Design review of the part built by this model. Coordinates are the model's own, in mm. Face numbers are marked on the shaded views. A direction names the side the tool comes from. Round coordinates to 2 decimals unless told otherwise and drop trailing zeros. Loops run counter-clockwise (first coordinate to the right, second up) from the corner with the lowest first, then second, coordinate; pieces in that order, holes last. Notation, with made-up numbers: (41.25, -33) -> (100.25, -33) arc R29 cw to (100.25, -8) -> close; hole circle Ø1 at (76.5, -1.5). An arc over 180 degrees is marked (long way). Answer as CSV lines item,"result". Start each with the question number.
(1) Machinability: for the marked faces 4, 5, 6, 7 and 8, which of the approach directions +Z, -Z, +X, -X, +Y, -Y give a long, thin tool a straight path to every point of the face, cutting with its end or side? Answer none if there is none.
(2) Take a section at C-C, the plane z = -15.5. Write out the cut boundary in (x, y), and give its area (4 significant figures).
(3) Draft analysis for pull direction Z (two halves, no side actions). For the marked faces 1, 2 and 3, state which applies: +Z half, -Z half, draft (parallel to the pull), parting line (faces both ways), or undercut.
(4) Take a section at A-A, the plane y = 54.5. Write out the cut boundary in (x, z), and give its area (3 significant figures).
(5) To check wall thickness, follow line 1 (Z direction, x = 24, y = 43); line 2 (X direction, y = 4, z = 28.5); line 3 (Z direction, x = 54, y = 28). State the ranges of each line that lie inside material, in increasing order. Write a range as from..to.
(6) For P1, Ø1, axis at x = 36.5, z = -16, coming from the +Y side; P2, Ø5, axis at x = 23, z = 7, coming from the -Y side; P3, Ø4, axis at x = 60.5, z = -24, coming from the +Y side, all flat-tipped, find the tip position at first contact; note any pin that passes through.
(7) Take a section at D-D, the plane y = 17. Write out the cut boundary in (x, z).
(8) Take a section at B-B, the plane x = 16.5. Write out the cut boundary in (y, z), and give its area (3 significant figures).
from build123d import *

# Parameters (mm, degrees)
BOSS_EXTRUDE1_DEPTH = 35
CUT_EXTRUDE1_DEPTH  = 10
SKETCH3_W           = 30
SKETCH3_H           = 15
CUT_EXTRUDE2_DEPTH  = 20


with BuildPart() as part:
    # Sketch1 → Boss-Extrude1 (new body, symmetric)
    with BuildSketch(Plane.XY):
        Polygon((0, 0), (0, 60), (15, 60), (40, 30), (80, 30), (80, 0), (60, 0), (60, 5), (20, 5), (20, 0), align=None)
    extrude(amount=BOSS_EXTRUDE1_DEPTH, both=True)

    # Sketch2 → Cut-Extrude1 (cut, symmetric)
    with BuildSketch(Plane.XY):
        Polygon((15, 60), (0, 60), (0, 40), (31.666666667, 40), align=None)
    extrude(amount=CUT_EXTRUDE1_DEPTH, both=True, mode=Mode.SUBTRACT)

    # Sketch3 → Cut-Extrude2 (cut, symmetric)
    with BuildSketch(Plane.XY):
        with Locations((65, 22.5)):
            Rectangle(SKETCH3_W, SKETCH3_H)
    extrude(amount=CUT_EXTRUDE2_DEPTH, both=True, mode=Mode.SUBTRACT)


solid = part.part
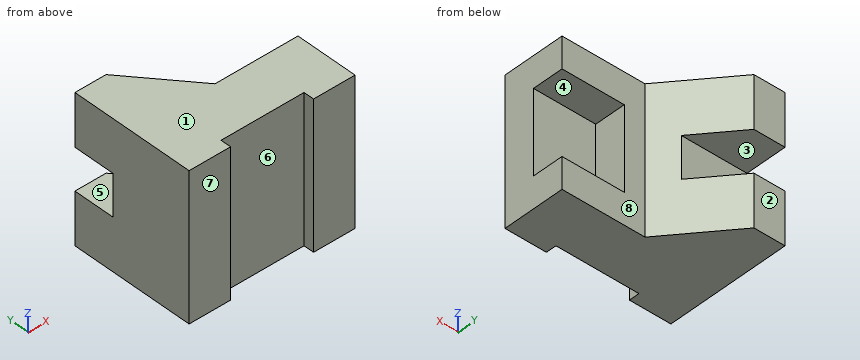
The answers:
1,face 4,"+X, +Y"
1,face 5,"+X, -X, +Y"
1,face 6,"+Z, -Z, -Y"
1,face 7,"+Z, -Z, +X, -X, -Y"
1,face 8,"+Z, -Z, +X, +Y"
2,outline,"(0, 0) -> (20, 0) -> (20, 5) -> (60, 5) -> (60, 0) -> (80, 0) -> (80, 15) -> (50, 15) -> (50, 30) -> (40, 30) -> (15, 60) -> (0, 60) -> close"
2,area,"2,575 mm²"
3,face 1,"+Z half"
3,face 2,"draft"
3,face 3,"undercut"
4,outline,"(0, -35) -> (19.58, -35) -> (19.58, -10) -> (0, -10) -> close; (0, 10) -> (19.58, 10) -> (19.58, 35) -> (0, 35) -> close"
4,area,"979 mm²"
5,line 1,"-35..-10, 10..35"
5,line 2,"0..20, 60..80"
5,line 3,"-35..-20, 20..35"
6,P1,"y = 34.8"
6,P2,"y = 5"
6,P3,"y = 30"
7,outline,"(0, -35) -> (80, -35) -> (80, -20) -> (50, -20) -> (50, 20) -> (80, 20) -> (80, 35) -> (0, 35) -> close"
8,outline,"(0, -35) -> (58.2, -35) -> (58.2, -10) -> (40, -10) -> (40, 10) -> (58.2, 10) -> (58.2, 35) -> (0, 35) -> close"
8,area,"3,710 mm²"
